Geometry check sheet. Reference: the model listing, model coordinates, mm. A direction names the side the tool comes from. Coordinates: 2 decimals unless noted, no trailing zeros. Write each loop counter-clockwise with the first axis right and the second up, starting at its lowest first coordinate (ties: lowest second). Pieces come first, ordered by that corner, then holes. Notation, with made-up numbers: (86, 79) -> (116, 79) arc R6 cw to (116, 89) -> close; hole circle Ø1 at (-19, -11.75). An arc over 180 degrees is marked (long way). Answer as CSV lines item,"result".
```python
from build123d import *

# Parameters (mm, degrees)
F0_W      = 50
F0_H      = 95
F1_DEPTH  = 40
F2_R      = 2.5
F3_DEPTH  = 18
F4_R      = 11.5
F5_DEPTH  = 20
F7_R      = 11.5
F8_DEPTH  = 50.001
F9_R      = 3
F10_DEPTH = 25


# Not quite as in the source:
# - a pattern or mirror of a feature is missing from the dataset's text; its kind, count and spacing are read off the source's solid


with BuildPart() as f1:
    # F0 (on Front) → F1 (new body)
    with BuildSketch(Plane.XZ):
        with Locations((25, 47.5)):
            Rectangle(F0_W, F0_H)
    extrude(amount=F1_DEPTH)

    # F2 (on face) → F3 (cut)
    with BuildSketch(Plane.XZ.offset(40)):
        with Locations((5, 5)):
            Circle(F2_R)
        with Locations((44.5, 5)):
            Circle(F2_R)
        with Locations((5, 45)):
            Circle(F2_R)
        with Locations((44.5, 45)):
            Circle(F2_R)
    extrude(amount=-F3_DEPTH, mode=Mode.SUBTRACT)

    # F4 (on face) → F5 (cut)
    with BuildSketch(Plane(origin=(0, 0, 0), x_dir=(0, -1, 0), z_dir=(-1, 0, 0))):
        with Locations((20, 74.5)):
            Circle(F4_R)
        with Locations((20, 20.5)):
            Circle(F4_R)
    f5 = extrude(amount=-F5_DEPTH, mode=Mode.SUBTRACT)

    # F5_copies: F5 across plane
    add(f5.mirror(Plane(origin=(25, 0, 0), x_dir=(0, 0, 1), z_dir=(1, 0, 0))), mode=Mode.SUBTRACT)

    # F7 (on face) → F8 (cut, through all)
    with BuildSketch(Plane(origin=(0, 0, 0), x_dir=(0, -1, 0), z_dir=(-1, 0, 0))):
        with Locations((20, 47.5)):
            Circle(F7_R)
    extrude(amount=-F8_DEPTH, mode=Mode.SUBTRACT)

    # F9 (on face) → F10 (cut)
    with BuildSketch(Plane(origin=(0, 0, 0), x_dir=(0, -1, 0), z_dir=(-1, 0, 0))):
        with Locations((32.5, 57.5)):
            Circle(F9_R)
        with Locations((7.5, 37.5)):
            Circle(F9_R)
    extrude(amount=-F10_DEPTH, mode=Mode.SUBTRACT)


solid = f1.part
```
Item 1: Cross-section at B-B, the plane z = 74.5. Record the cut outline in (x, y).
Responses:
outline,"(0, -40) -> (50, -40) -> (50, -31.5) -> (30, -31.5) -> (30, -8.5) -> (50, -8.5) -> (50, 0) -> (0, 0) -> (0, -8.5) -> (20, -8.5) -> (20, -31.5) -> (0, -31.5) -> close"
Item 2: Cross-section at C-C, the plane x = 44.5. Record the cut outline in (y, z).
Responses:
outline,"(-40, 0) -> (0, 0) -> (0, 95) -> (-40, 95) -> (-40, 47.5) -> (-31.5, 47.5) arc R11.5 cw (long way) to (-30.36, 42.5) -> (-40, 42.5) -> (-40, 7.5) -> (-22, 7.5) -> (-22, 2.5) -> (-40, 2.5) -> close; hole circle Ø23 at (-20, 20.5); hole circle Ø23 at (-20, 74.5)"
Item 3: Thickness scan on probe 1 along Z at (x, y) = (44.5, -34.75); probe 2 along Y at (x, z) = (7, 74); probe 3 along Z at (x, y) = (5, -32). Record the ranges inside material, lowest first.
Responses:
probe 1,"z = 0 to 2.5, 7.5 to 42.5, 47.5 to 95"
probe 2,"y = -40 to -31.49, -8.51 to 0"
probe 3,"z = 0 to 2.5, 7.5 to 42.5, 47.5 to 54.54, 60.46 to 95"
Item 4: Cross-section at D-D, the plane y = -7.5. Record the cut outline in (x, z), plus the area to 3 significant figures.
Responses:
outline,"(0, 0) -> (50, 0) -> (50, 95) -> (0, 95) -> (0, 40.5) -> (25, 40.5) -> (25, 34.5) -> (0, 34.5) -> close"
area,"4,600 mm2"
Item 5: Cross-section at A-A, the plane y = -20. Record the cut outline in (x, z).
Responses:
outline,"(0, 0) -> (50, 0) -> (50, 9) -> (30, 9) -> (30, 32) -> (50, 32) -> (50, 36) -> (0, 36) -> (0, 32) -> (20, 32) -> (20, 9) -> (0, 9) -> close; (0, 59) -> (50, 59) -> (50, 63) -> (30, 63) -> (30, 86) -> (50, 86) -> (50, 95) -> (0, 95) -> (0, 86) -> (20, 86) -> (20, 63) -> (0, 63) -> close"
Item 6: Release check for a two-part mould opening along Y. For faces 6 (the cylindrical face through (9.86, -30.97, 23.95)), 7 (the flat face through (25, -20, 0)), 8 (the flat face through (25, -40, 48)) record: +Y half, -Y half, draft (parallel to the pull), parting line (faces both ways), or undercut.
Responses:
face 6,"undercut"
face 7,"draft"
face 8,"-Y half"
Item 7: Set-up check for faces 1 (the flat face through (20, -20, 21)), 2 (the flat face through (0, -15, 36)), 3 (the flat face through (44, -22, 5)), 4 (the flat face through (25, -20, 95)), 5 (the flat face through (30, -20, 75)): record each of +Z, -Z, +X, -X, +Y, -Y from which the full face is reachable in a straight line by a thin tool's end or side.
Responses:
face 1,"-X"
face 2,"+Z, -Z, -X, +Y, -Y"
face 3,"-Y"
face 4,"+Z, +X, -X, +Y, -Y"
face 5,"+X"
Item 8: Depth check by flat-ended pin: pin 1 Ø18.5 at (y, z) = (-23.5, 21) entering from -X; pin 2 Ø5 at (y, z) = (-32.5, 57.5) entering from -X; pin 3 Ø4.5 at (x, z) = (5, 5) entering from -Y; pin 4 Ø14 at (y, z) = (-20, 74.5) entering from -X. Enter the tip coordinate at first touch or a pass-through.
Responses:
pin 1,"stops at x = 0"
pin 2,"stops at x = 25"
pin 3,"stops at y = -22"
pin 4,"stops at x = 20"
